Build history of the part. All positions in model axes, mm. Round coordinates to 2 decimals unless told otherwise and drop trailing zeros. Order: outer loops, then holes, each group sorted by start corner. A loop starts at its lowest first (then second) coordinate and runs counter-clockwise, first axis right, second up. Notation, with made-up numbers: (-12, 3) -> (-1, 3) arc R29 cw to (-1, 41) -> close; hole circle Ø2 at (30.5, 61.5). An arc over 180 degrees is marked (long way). Answer as a JSON object with one key per item and string values.
Autodesk Inventor part; units mm, degrees
ref_plane "YZ Plane" through (0, 0, 0) normal (1, 0, 0) x (0, 1, 0)
ref_plane "XZ Plane" through (0, 0, 0) normal (0, 1, 0) x (-1, 0, 0)
ref_plane "XY Plane" through (0, 0, 0) normal (0, 0, 1) x (1, 0, 0)
sketch "スケッチ1" plane through (0, 0, 0) normal (0, 0, 1) x (1, 0, 0)
  line L0 (9.406, -6.0438) -> (-42.1785, -36.6875)
  line L1 (-42.1785, -36.6875) -> (-83.0369, 32.0918)
  line L2 (-83.0369, 32.0918) -> (-31.4524, 62.7355)
  line L3 (-31.4524, 62.7355) -> (9.406, -6.0438)
  circle A0 centre (-42.9871, -25.5365) radius 1.3
  circle A1 centre (-74.7819, 27.9857) radius 1.3
  circle A2 centre (-30.6438, 51.5845) radius 1.3
  circle A3 centre (0, 0) radius 1.3
  line L4 (-30.6438, 51.5845) -> (-26.3451, 54.1381) construction
  line L5 (-30.6438, 51.5845) -> (-35.7511, 60.1819) construction
  line L6 (-42.9871, -25.5365) -> (-47.2858, -28.0901) construction
  line L7 (-42.9871, -25.5365) -> (-37.8798, -34.1339) construction
  line L8 (-74.7819, 27.9857) -> (-78.7381, 34.6454) construction
  line L9 (-74.7819, 27.9857) -> (-79.0806, 25.432) construction
  line L10 (0, 0) -> (4.2987, 2.5536) construction
  line L11 (0, 0) -> (5.1073, -8.5974) construction
  point P0 (0, 0)
  dimension "d2" = 80
  dimension "d3" = 60
extrude "押し出し1" add sketch "スケッチ1" along normal blind 1
properties part number "ThirdPlate"
1) Pull direction X, two halves, no side cores. Call faces 1 (the face through (-30.813, 50.296, 0.493)), 2 (the face through (-0.17, -1.29, 0.49)), 3 (the face through (-62.32, -2.78, 0.49)), 4 (the face through (-16.025, -21.151, 0.493)): pulls with the +X half, pulls with the -X half, needs draft (parallel to the pull), parting line crosses it, or undercut.
Checked values:
{"face 1": "undercut", "face 2": "undercut", "face 3": "pulls with the -X half", "face 4": "pulls with the +X half"}
2) Cut at B-B, the plane x = 0. Give the cut face in (y, z).
Checked values:
{"outline": "(-11.63, 0) -> (-1.3, 0) -> (-1.3, 1) -> (-11.63, 1) -> close; (1.3, 0) -> (9.79, 0) -> (9.79, 1) -> (1.3, 1) -> close"}
3) Cut at D-D, the plane x = -37.5. Give the cut face in (y, z).
Checked values:
{"outline": "(-33.91, 0) -> (59.14, 0) -> (59.14, 1) -> (-33.91, 1) -> close"}
4) Cut at A-A, the plane y = 0. Give the cut face in (x, z).
Checked values:
{"outline": "(-63.97, 0) -> (-1.3, 0) -> (-1.3, 1) -> (-63.97, 1) -> close; (1.3, 0) -> (5.82, 0) -> (5.82, 1) -> (1.3, 1) -> close"}
5) Flat gauge pin, fed straight in: pin 1 Ø2.5 at (x, y) = (-42.99, -25.54) entering from +Z. Where does the tip first touch, or does it go through?
Checked values:
{"pin 1": "passes through"}
6) Probe L1, parallel to Y at x = -74.5, z = 0.4; L2, parallel to Y at x = 0, z = 0.8; L3, parallel to Y at x = -49.5, z = 0.1. List the from-to ranges inside material, lowest first. Write a range as from..to.
Checked values:
{"L1": "y = 17.72..26.72, 29.25..37.16", "L2": "y = -11.63..-1.3, 1.3..9.79", "L3": "y = -24.36..52.01"}
7) Cut at C-C, the plane z = 0.4. Give the cut face in (x, y), plus the area to 3 significant figures.
Checked values:
{"outline": "(-83.04, 32.09) -> (-42.18, -36.69) -> (9.41, -6.04) -> (-31.45, 62.74) -> close; hole circle Ø2.6 at (-74.78, 27.99); hole circle Ø2.6 at (-42.99, -25.54); hole circle Ø2.6 at (-30.64, 51.58); hole circle Ø2.6 at (0, 0)", "area": "4,780 mm²"}
